Could you check a few things on this model? Use its own coordinates, in mm. Give positions to 0.01 mm unless a question says otherwise; leave off trailing zeros. Loops run counter-clockwise (first coordinate to the right, second up) from the corner with the lowest first, then second, coordinate; pieces in that order, holes last. Notation, with made-up numbers: M -34.75,-21.75 L -18.75,-21.75 A7 cw -18.75,-15.75 Z; hole C -5,20.25 d2. An arc over 180 degrees is marked long. Use a Markdown table: item, result. Add a question column.
1) Will these pins go through, and if not, where does the flat tip stop? pin 1 Ø6 at (y, z) = (-7, -4) entering from +X; pin 2 Ø6 at (y, z) = (-20.5, 1.5) entering from -X; pin 3 Ø1.5 at (y, z) = (-22.5, -2) entering from +X; pin 4 Ø2 at (x, z) = (5, -3.5) entering from +Y.
2) If I drill on line 1 along Y through (x, z) = (-0.5, -0.25); line 2 along X through (y, z) = (-7.5, -0.25) (3 decimals); line 3 along X through (y, z) = (3.5, -3), over which ranges is the centre line in solid material (lowest first)? Write a range as [from, to].
3) Suppose I cut it at A-A on y = -6. List the corners of the cut face in (x, z) for me.
Autodesk Inventor part; units mm, degrees
ref_plane "YZ Plane" through (0, 0, 0) normal (1, 0, 0) x (0, 1, 0)
ref_plane "XZ Plane" through (0, 0, 0) normal (0, 1, 0) x (-1, 0, 0)
ref_plane "XY Plane" through (0, 0, 0) normal (0, 0, 1) x (1, 0, 0)
sketch "Sketch1" plane through (0, 0, 0) normal (0, 0, 1) x (1, 0, 0)
  line L0 (0, 5.3298) -> (6.25, 5.3298)
  line L1 (6.25, -14.6702) -> (0, -14.6702)
  line L2 (0, -14.6702) -> (0, 5.3298)
  circle A0 centre (6.25, -9.5902) radius 0.635
  line L3 (6.25, 5.3298) -> (6.25, -8.9552)
  line L4 (6.25, -10.2252) -> (6.25, -14.6702)
  point P0 (0, 0)
  dimension "d0" = 6.25
  dimension "d1" = 20
  dimension "d2" = 1.27
  dimension "d3" = 5.08
revolve "Revolution1" add sketch "Sketch1" angle 360 about axis through (0, -14.6702, 0) along (0, 1, 0) contours L0 L3 A0 L4 L1 L2
fillet "Fillet1" radius 0.508 3 edges at (-6.25, -10.2252, 0) (-6.25, -8.9552, 0) (-6.25, 5.3298, 0)
sketch "Sketch2" plane through (0, -14.6702, 0) normal (0, -1, 0) x (1, 0, 0)
  circle A0 centre (0, 2.5) radius 0.3
  circle A1 centre (0, -2.5) radius 0.3
  point P0 (0, 0)
  dimension "d6" = 0.6
  dimension "d7" = 0.6
  dimension "d8" = 2.5
  dimension "d9" = 2.5
extrude "Extrusion1" add sketch "Sketch2" along normal blind 15
sketch "Sketch3" plane through (0, -29.6702, -2.5) normal (0, -1, 0) x (1, 0, 0)
  circle A0 centre (0, 0) radius 0.3
  point P0 (0, 2.5)
extrude "Extrusion2" add sketch "Sketch3" along normal blind 4
equation "\"d7\" = d6"
properties part number "CAP12.5X20" material "PC/ABS Plastic"
Answer block:
| question | item | result |
|---|---|---|
| 1 | pin 1 | stops at x = 6.17 |
| 1 | pin 2 | stops at x = -0.3 |
| 1 | pin 3 | stops at x = 0.3 |
| 1 | pin 4 | stops at y = 5.33 |
| 2 | line 1 | y = [-14.67, 5.33] |
| 2 | line 2 | x = [-6.245, 6.245] |
| 2 | line 3 | x = [-5.48, 5.48] |
| 3 | outline | C 0,0 d12.5 |
